from build123d import *

# Parameters (mm, degrees)
EXTRUDE_1_DEPTH          = 297
SKETCH_6_R               = 57.15
CUT_EXTRUDE_1_DEPTH      = 5
CUT_EXTRUDE_2_REACH      = 528.789
SKETCH_7_R               = 26
CUT_EXTRUDE_3_REACH      = 530.764
SKETCH_8_R               = 58
CUT_EXTRUDE_4_REACH      = 521.294
SKETCH_10_R              = 5.5
HOLE_WIZARD_M12_1_D      = 13.5
HOLE_WIZARD_M12_1_DEPTH  = 25
PATTERN_CIRCULAR_1_COUNT = 4


with BuildPart() as part:
    # 草图4 → 凸台-拉伸1 (new body)
    with BuildSketch(Plane(origin=(0, 0, 0), x_dir=(1, 0, 0), z_dir=(0, 1, 0))):
        Polygon((-258.320541352, -83.224920734), (-258.320541352, -53.224920734), (-233.320541352, -53.224920734), (-233.320541352, -383.224920734), (-258.320541352, -383.224920734), (-258.320541352, -353.224920734), (-444.320541352, -353.224920734), (-444.320541352, -83.224920734), align=None)
        with BuildLine():
            Line((-258.320541352, -313.224920734), (-258.320541352, -123.224920734))
            ThreePointArc((-258.320541352, -123.224920734), (-264.178405729, -109.08278511), (-278.320541352, -103.224920734))
            Line((-278.320541352, -103.224920734), (-399.320541352, -103.224920734))
            ThreePointArc((-399.320541352, -103.224920734), (-413.462676976, -109.08278511), (-419.320541352, -123.224920734))
            Line((-419.320541352, -123.224920734), (-419.320541352, -313.224920734))
            ThreePointArc((-419.320541352, -313.224920734), (-413.462676976, -327.367056358), (-399.320541352, -333.224920734))
            Line((-399.320541352, -333.224920734), (-278.320541352, -333.224920734))
            ThreePointArc((-278.320541352, -333.224920734), (-264.178405729, -327.367056358), (-258.320541352, -313.224920734))
        make_face(mode=Mode.SUBTRACT)
    extrude(amount=EXTRUDE_1_DEPTH)

    # 草图6 → 切除-拉伸1 (cut)
    with BuildSketch(Plane.ZY.offset(444.320541352)):
        with Locations((218.224920734, 202)):
            Circle(SKETCH_6_R)
    extrude(amount=-CUT_EXTRUDE_1_DEPTH, mode=Mode.SUBTRACT)

    # 草图7 → 切除-拉伸2 (cut, up to next)
    with BuildSketch(Plane.ZY.offset(439.320541352), mode=Mode.PRIVATE) as cut_extrude_2_sk1:
        with Locations((218.224920734, 202)):
            Circle(SKETCH_7_R)
    cut_extrude_2_tool1 = extrude(cut_extrude_2_sk1.sketch, amount=-CUT_EXTRUDE_2_REACH, mode=Mode.PRIVATE) & part.part
    add(cut_extrude_2_tool1.solids().sort_by_distance((-439.320541, 202, 218.224921))[0], mode=Mode.SUBTRACT)

    # 草图8 → 切除-拉伸3 (cut, up to next)
    with BuildSketch(Plane(origin=(-233.320541352, 0, 0), x_dir=(0, 0, -1), z_dir=(1, 0, 0)), mode=Mode.PRIVATE) as cut_extrude_3_sk1:
        with Locations((-218.224920734, 202)):
            Circle(SKETCH_8_R)
    cut_extrude_3_tool1 = extrude(cut_extrude_3_sk1.sketch, amount=-CUT_EXTRUDE_3_REACH, mode=Mode.PRIVATE) & part.part
    add(cut_extrude_3_tool1.solids().sort_by_distance((-233.320541, 202, 218.224921))[0], mode=Mode.SUBTRACT)

    # 草图10 → 切除-拉伸4 (cut, up to next)
    with BuildSketch(Plane.ZY.offset(258.320541352), mode=Mode.PRIVATE) as cut_extrude_4_sk1:
        with Locations((368.224920734, 15)):
            Circle(SKETCH_10_R)
    cut_extrude_4_tool1 = extrude(cut_extrude_4_sk1.sketch, amount=-CUT_EXTRUDE_4_REACH, mode=Mode.PRIVATE) & part.part
    # 草图10 → 切除-拉伸4 (cut, up to next)
    with BuildSketch(Plane.ZY.offset(258.320541352), mode=Mode.PRIVATE) as cut_extrude_4_sk2:
        with Locations((368.224920734, 57)):
            Circle(SKETCH_10_R)
    cut_extrude_4_tool2 = extrude(cut_extrude_4_sk2.sketch, amount=-CUT_EXTRUDE_4_REACH, mode=Mode.PRIVATE) & part.part
    # 草图10 → 切除-拉伸4 (cut, up to next)
    with BuildSketch(Plane.ZY.offset(258.320541352), mode=Mode.PRIVATE) as cut_extrude_4_sk3:
        with Locations((368.224920734, 99)):
            Circle(SKETCH_10_R)
    cut_extrude_4_tool3 = extrude(cut_extrude_4_sk3.sketch, amount=-CUT_EXTRUDE_4_REACH, mode=Mode.PRIVATE) & part.part
    # 草图10 → 切除-拉伸4 (cut, up to next)
    with BuildSketch(Plane.ZY.offset(258.320541352), mode=Mode.PRIVATE) as cut_extrude_4_sk4:
        with Locations((368.224920734, 141)):
            Circle(SKETCH_10_R)
    cut_extrude_4_tool4 = extrude(cut_extrude_4_sk4.sketch, amount=-CUT_EXTRUDE_4_REACH, mode=Mode.PRIVATE) & part.part
    # 草图10 → 切除-拉伸4 (cut, up to next)
    with BuildSketch(Plane.ZY.offset(258.320541352), mode=Mode.PRIVATE) as cut_extrude_4_sk5:
        with Locations((68.224920734, 141)):
            Circle(SKETCH_10_R)
    cut_extrude_4_tool5 = extrude(cut_extrude_4_sk5.sketch, amount=-CUT_EXTRUDE_4_REACH, mode=Mode.PRIVATE) & part.part
    # 草图10 → 切除-拉伸4 (cut, up to next)
    with BuildSketch(Plane.ZY.offset(258.320541352), mode=Mode.PRIVATE) as cut_extrude_4_sk6:
        with Locations((68.224920734, 15)):
            Circle(SKETCH_10_R)
    cut_extrude_4_tool6 = extrude(cut_extrude_4_sk6.sketch, amount=-CUT_EXTRUDE_4_REACH, mode=Mode.PRIVATE) & part.part
    # 草图10 → 切除-拉伸4 (cut, up to next)
    with BuildSketch(Plane.ZY.offset(258.320541352), mode=Mode.PRIVATE) as cut_extrude_4_sk7:
        with Locations((68.224920734, 57)):
            Circle(SKETCH_10_R)
    cut_extrude_4_tool7 = extrude(cut_extrude_4_sk7.sketch, amount=-CUT_EXTRUDE_4_REACH, mode=Mode.PRIVATE) & part.part
    # 草图10 → 切除-拉伸4 (cut, up to next)
    with BuildSketch(Plane.ZY.offset(258.320541352), mode=Mode.PRIVATE) as cut_extrude_4_sk8:
        with Locations((68.224920734, 99)):
            Circle(SKETCH_10_R)
    cut_extrude_4_tool8 = extrude(cut_extrude_4_sk8.sketch, amount=-CUT_EXTRUDE_4_REACH, mode=Mode.PRIVATE) & part.part
    add(cut_extrude_4_tool1.solids().sort_by_distance((-258.320541, 15, 368.224921))[0], mode=Mode.SUBTRACT)
    add(cut_extrude_4_tool2.solids().sort_by_distance((-258.320541, 57, 368.224921))[0], mode=Mode.SUBTRACT)
    add(cut_extrude_4_tool3.solids().sort_by_distance((-258.320541, 99, 368.224921))[0], mode=Mode.SUBTRACT)
    add(cut_extrude_4_tool4.solids().sort_by_distance((-258.320541, 141, 368.224921))[0], mode=Mode.SUBTRACT)
    add(cut_extrude_4_tool5.solids().sort_by_distance((-258.320541, 141, 68.224921))[0], mode=Mode.SUBTRACT)
    add(cut_extrude_4_tool6.solids().sort_by_distance((-258.320541, 15, 68.224921))[0], mode=Mode.SUBTRACT)
    add(cut_extrude_4_tool7.solids().sort_by_distance((-258.320541, 57, 68.224921))[0], mode=Mode.SUBTRACT)
    add(cut_extrude_4_tool8.solids().sort_by_distance((-258.320541, 99, 68.224921))[0], mode=Mode.SUBTRACT)

    # M12 间隙孔1
    with Locations(Plane.ZY.offset(444.320541352)):
        with Locations((147.514920734, 272.711356231)):
            hole_wizard_m12_1 = Hole(HOLE_WIZARD_M12_1_D / 2, depth=HOLE_WIZARD_M12_1_DEPTH)

    # 阵列(圆周)1: M12 间隙孔1 ×4 about axis
    pattern_circular_1_axis = Axis((0, 202, 218.224920734), (1, 0, 0))
    for i in range(1, PATTERN_CIRCULAR_1_COUNT):
        add(hole_wizard_m12_1.rotate(pattern_circular_1_axis, i * 360 / PATTERN_CIRCULAR_1_COUNT), mode=Mode.SUBTRACT)


solid = part.part
Verification items for the finished model (mm, model axes). A direction names the side the tool comes from. Coordinates: 2 decimals unless noted, no trailing zeros. Loops run counter-clockwise (first coordinate to the right, second up) from the corner with the lowest first, then second, coordinate; pieces in that order, holes last. Notation, with made-up numbers: (83, 74) -> (118, 74) arc R29 ccw to (118, 113) -> close; hole circle Ø8 at (2.25, 86.25). An arc over 180 degrees is marked (long way). Answer as a JSON object with one key per item and string values. Group by question number.
Item 1: Sectioned sample at A-A on x = -336.5. Record the boundary of the cut face in (y, z), plus the area to 3 significant figures.
Item 2: Mould release check, pull along Z, two halves, no side actions. Record for faces 1 (the cylindrical face through (-431.646, 138.033, 147.217)), 2 (the flat face through (-246, 146, 383.225)), 3 (the flat face through (-233.321, 113, 216)): +Z half, -Z half, draft (parallel to the pull), parting line (faces both ways), or undercut.
Item 3: Scan lines: probe 1 along X at (y, z) = (146, 193.5); probe 2 along Z at (x, y) = (-281.5, 54.5); probe 3 along Z at (x, y) = (-277, 114.5). Record each from-to range of solid material in increasing order.
Item 4: Sectioned sample at B-B on y = 57. Record the boundary of the cut face in (x, z), plus the area to 3 significant figures.
Item 5: Tool access check on faces 4 (the flat face through (-258.321, 146, 365)), 5 (the flat face through (-258.321, 146, 72)), 6 (the cylindrical face through (-245.646, 179.786, 164.648)), 7 (the flat face through (-340, 146, 333.225)), 8 (the cylindrical face through (-431.646, 265.967, 289.233)). Record the directions out of +Z, -Z, +X, -X, +Y, -Y that give a thin tool (end or side, any length) a straight path to the whole face; none if there is none.
Item 6: Sectioned sample at D-D on z = 227.5. Record the boundary of the cut face in (x, y), plus the area to 3 significant figures.
Item 7: Sectioned sample at C-C on y = 202. Record the boundary of the cut face in (x, z), plus the area to 3 significant figures.
Item 8: Depth check by flat-ended pin: pin 1 (12 mm diameter, centred on x = -375, y = 199, fed in from -Z); pin 2 (17.5 mm diameter, centred on y = 99, z = 68.22, fed in from -X); pin 3 (6 mm diameter, centred on x = -320, y = 32.5, fed in from +Z). Enter the tip coordinate at first touch or a pass-through.
Evaluation:
{
 "1": {"outline": "(0, 83.22) -> (297, 83.22) -> (297, 103.22) -> (0, 103.22) -> close; (0, 333.22) -> (297, 333.22) -> (297, 353.22) -> (0, 353.22) -> close", "area": "11,900 mm²"},
 "2": {"face 1": "undercut", "face 2": "+Z half", "face 3": "draft"},
 "3": {"probe 1": "x = -444.32 to -419.32, -258.32 to -233.32", "probe 2": "z = 83.22 to 103.22, 333.22 to 353.22", "probe 3": "z = 83.22 to 103.27, 333.18 to 353.22"},
 "4": {"outline": "(-444.32, 83.22) -> (-258.32, 83.22) -> (-258.32, 73.72) -> (-233.32, 73.72) -> (-233.32, 362.72) -> (-258.32, 362.72) -> (-258.32, 353.22) -> (-444.32, 353.22) -> close; (-258.32, 53.22) -> (-233.32, 53.22) -> (-233.32, 62.72) -> (-258.32, 62.72) -> close; (-258.32, 373.72) -> (-233.32, 373.72) -> (-233.32, 383.22) -> (-258.32, 383.22) -> close; hole (-419.32, 123.22) arc R20 ccw to (-399.32, 103.22) -> (-278.32, 103.22) arc R20 ccw to (-258.32, 123.22) -> (-258.32, 313.22) arc R20 ccw to (-278.32, 333.22) -> (-399.32, 333.22) arc R20 ccw to (-419.32, 313.22) -> close", "area": "21,200 mm²"},
 "5": {"face 4": "+Z, -X, +Y, -Y", "face 5": "-Z, -X, +Y, -Y", "face 6": "+X", "face 7": "+Y, -Y", "face 8": "-X"},
 "6": {"outline": "(-444.32, 0) -> (-419.32, 0) -> (-419.32, 177.71) -> (-439.32, 177.71) -> (-439.32, 145.61) -> (-444.32, 145.61) -> close; (-444.32, 258.39) -> (-439.32, 258.39) -> (-439.32, 226.29) -> (-419.32, 226.29) -> (-419.32, 297) -> (-444.32, 297) -> close; (-258.32, 0) -> (-233.32, 0) -> (-233.32, 144.75) -> (-258.32, 144.75) -> close; (-258.32, 259.25) -> (-233.32, 259.25) -> (-233.32, 297) -> (-258.32, 297) -> close", "area": "10,500 mm²"},
 "7": {"outline": "(-444.32, 83.22) -> (-258.32, 83.22) -> (-258.32, 53.22) -> (-233.32, 53.22) -> (-233.32, 160.22) -> (-258.32, 160.22) -> (-258.32, 123.22) arc R20 cw to (-278.32, 103.22) -> (-399.32, 103.22) arc R20 cw to (-419.32, 123.22) -> (-419.32, 192.22) -> (-439.32, 192.22) -> (-439.32, 161.07) -> (-444.32, 161.07) -> close; (-444.32, 275.37) -> (-439.32, 275.37) -> (-439.32, 244.22) -> (-419.32, 244.22) -> (-419.32, 313.22) arc R20 cw to (-399.32, 333.22) -> (-278.32, 333.22) arc R20 cw to (-258.32, 313.22) -> (-258.32, 276.22) -> (-233.32, 276.22) -> (-233.32, 383.22) -> (-258.32, 383.22) -> (-258.32, 353.22) -> (-444.32, 353.22) -> close", "area": "17,300 mm²"},
 "8": {"pin 1": "stops at z = 83.22", "pin 2": "stops at x = -258.32", "pin 3": "stops at z = 353.22"}
}
